Input: dimensioned drawing with shaded views. Units: mm. Origin: part minimum x, y, z. Coordinates: 2 decimals unless noted, no trailing zeros. Loops run counter-clockwise (first coordinate to the right, second up) from the corner with the lowest first, then second, coordinate; pieces in that order, holes last. Notation, with made-up numbers: (56, 83) -> (68, 83) arc R28 cw to (68, 116) -> close; hole circle Ø6 at (2, 28.5). An arc over 180 degrees is marked (long way). Answer as CSV lines item,"result".
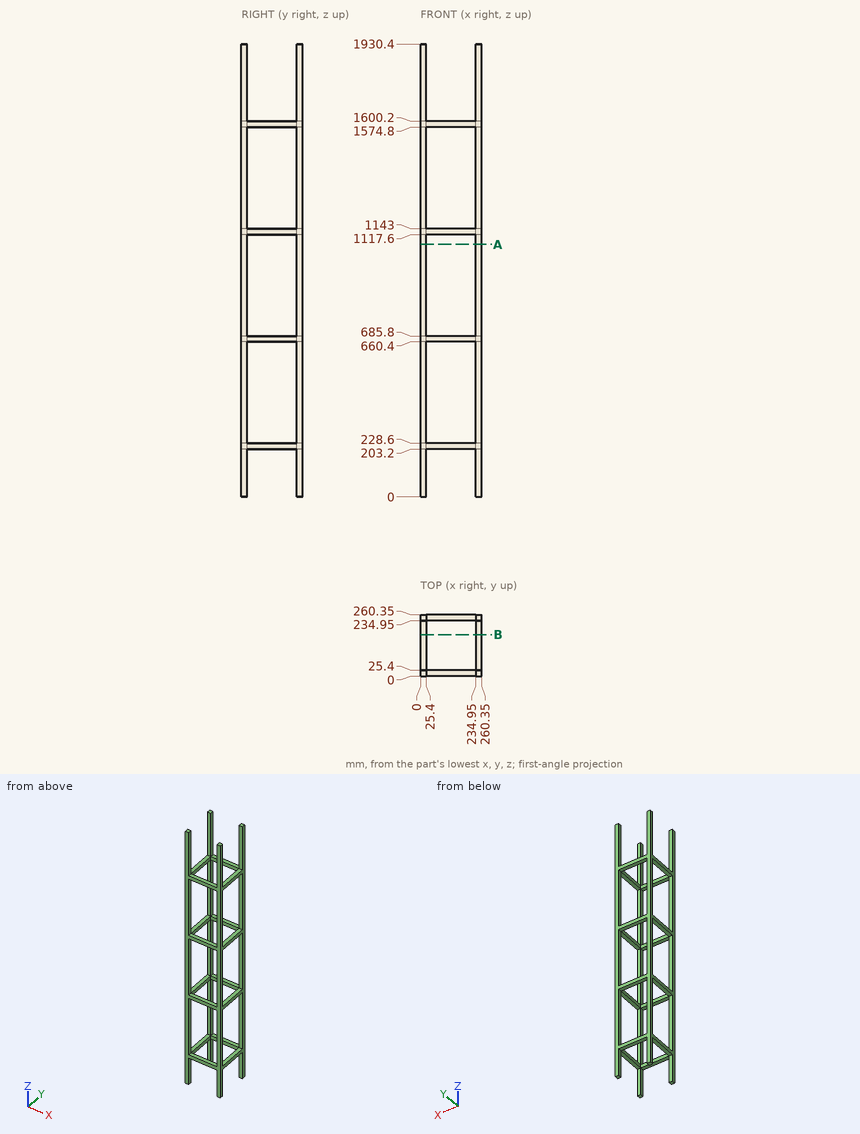
(1) Material intervals for L1, parallel to Z at x = 96.5, y = 246; L2, parallel to Y at x = 243.5, z = 381.5, sorted ascending. Write a range as [from, to].
Computed values:
L1,"[203.2, 228.6], [660.4, 685.8], [1117.6, 1143], [1574.8, 1600.2]"
L2,"[0, 25.4], [234.95, 260.35]"
(2) Pin query (flat end, axial travel): pin 1 Ø20.5 at (x, y) = (250, 126.5) entering from -Z. Return the tip coordinate at first contact, or that it passes through.
Computed values:
pin 1,"z = 203.2"
(3) Cut plane A-A (z = 1076). Return the cut outline in (x, y).
Computed values:
outline,"(0, 0) -> (25.4, 0) -> (25.4, 25.4) -> (0, 25.4) -> close; (0, 234.95) -> (25.4, 234.95) -> (25.4, 260.35) -> (0, 260.35) -> close; (234.95, 0) -> (260.35, 0) -> (260.35, 25.4) -> (234.95, 25.4) -> close; (234.95, 234.95) -> (260.35, 234.95) -> (260.35, 260.35) -> (234.95, 260.35) -> close"
(4) Cut plane B-B (y = 176). State how many separate pieces and enclosed holes the cut face has, then the cut area to 3 significant figures.
Computed values:
separate pieces,"8"
enclosed holes,"0"
area,"5,160 mm^2"
